Check sheet for the modelled part. Datum: model origin and axes. Units: mm. Round coordinates to 2 decimals unless told otherwise and drop trailing zeros. Order: outer loops, then holes, each group sorted by start corner. A loop starts at its lowest first (then second) coordinate and runs counter-clockwise, first axis right, second up.
```python
from build123d import *

# Parameters (mm, degrees)
SKETCH1_W                    = 220
SKETCH1_H                    = 560
BASE_FLANGE1_DEPTH           = 1.2
EDGE_FLANGE1_STRIP_W         = 8.2
EDGE_FLANGE1_STRIP_H         = 1.2
EDGE_FLANGE1_STRIP_CUT_DEPTH = 202.5
EDGE_FLANGE1_DEPTH           = 202.5
FILLET1_R                    = 1.5
SKETCH6_R                    = 2
CUT_EXTRUDE1_DEPTH           = 10
CUT_EXTRUDE2_DEPTH           = 10
LPATTERN1_COUNT              = 15
LPATTERN1_PITCH              = 7.2
FILLET2_R                    = 1.5


# Sheet-metal steps are written as plain solids
with BuildPart() as part:
    # Sketch1 → Base-Flange1 (new body)
    with BuildSketch(Plane(origin=(0, 0, 0), x_dir=(1, 0, 0), z_dir=(0, 1, 0))):
        with Locations((110, 280)):
            Rectangle(SKETCH1_W, SKETCH1_H)
    extrude(amount=BASE_FLANGE1_DEPTH)

    # Edge-Flange1 strip (across the edge) → Edge-Flange1 strip cut (cut)
    with BuildSketch(Plane(origin=(202.5, 0, 0), x_dir=(0, 0, -1), z_dir=(-1, 0, 0))):
        with Locations((-1.2, -0.6)):
            Rectangle(EDGE_FLANGE1_STRIP_W, EDGE_FLANGE1_STRIP_H)
    extrude(amount=EDGE_FLANGE1_STRIP_CUT_DEPTH, mode=Mode.SUBTRACT)

    # Edge-Flange1 section (across the edge) → Edge-Flange1 (add)
    with BuildSketch(Plane(origin=(202.5, 0, 0), x_dir=(0, 0, -1), z_dir=(-1, 0, 0))):
        with BuildLine():
            Line((0, 1.7), (0, 6.3))
            Line((0, 6.3), (1.2, 6.3))
            Line((1.2, 6.3), (1.2, 1.7))
            ThreePointArc((1.2, 1.7), (1.697918472, 0.497918472), (2.9, 0))
            Line((2.9, 0), (2.9, -1.2))
            ThreePointArc((2.9, -1.2), (0.849390335, -0.350609665), (0, 1.7))
        make_face()
    extrude(amount=EDGE_FLANGE1_DEPTH)

    # Fillet1
    fillet1_edges = [part.edges().sort_by_distance(p)[0] for p in [
        (202.5, -6.3, -0.6),
    ]]
    fillet(fillet1_edges, radius=FILLET1_R)

    # Sketch6 → Cut-Extrude1 (cut)
    with BuildSketch(Plane(origin=(0, 1.2, 0), x_dir=(1, 0, 0), z_dir=(0, 1, 0))):
        with Locations(Location((215.5, 531, 0), (0, 0, 270))):
            Circle(SKETCH6_R)
        with Locations(Location((215.5, 30, 0), (0, 0, 270))):
            Circle(SKETCH6_R)
        with Locations(Location((140, 555.5, 0), (0, 0, 270))):
            Circle(SKETCH6_R)
    extrude(amount=-CUT_EXTRUDE1_DEPTH, mode=Mode.SUBTRACT)

    # Sketch7 → Cut-Extrude2 (cut)
    with BuildSketch(Plane(origin=(0, 1.2, 0), x_dir=(1, 0, 0), z_dir=(0, 1, 0))):
        with BuildLine():
            Line((172.5, 477.1), (172.5, 512.9))
            ThreePointArc((172.5, 512.9), (174.6, 515), (176.7, 512.9))
            Line((176.7, 512.9), (176.7, 477.1))
            ThreePointArc((176.7, 477.1), (174.6, 475), (172.5, 477.1))
        make_face()
    cut_extrude2 = extrude(amount=-CUT_EXTRUDE2_DEPTH, mode=Mode.SUBTRACT)

    # LPattern1: Cut-Extrude2 ×15
    with Locations(*[(-i * LPATTERN1_PITCH, 0, 0) for i in range(1, LPATTERN1_COUNT)]):
        add(cut_extrude2, mode=Mode.SUBTRACT)

    # Fillet2
    fillet2_edges = [part.edges().sort_by_distance(p)[0] for p in [
        (220, 0.6, -560),
        (220, 0.6, 0),
    ]]
    fillet(fillet2_edges, radius=FILLET2_R)

    # Mirror1: part across plane


with BuildPart() as part_1:
    add(part.part)
    add(part.part.mirror(Plane(origin=(0, 1.2, 0), x_dir=(0, 0, 1), z_dir=(1, 0, 0))))


solid = part_1.part
```
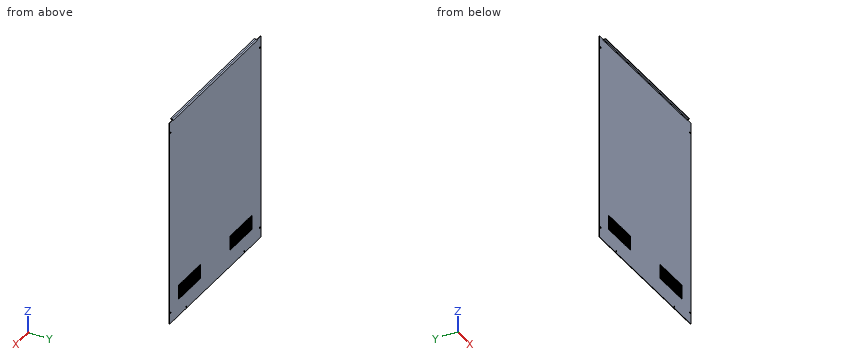
Item 1: Scan lines: line 1 along X through (y, z) = (0.45, -531); line 2 along Z through (x, y) = (-215.5, 0.4); line 3 along Z through (x, y) = (-140, 0.3). Record each from-to range of solid material in increasing order.
Answer:
line 1: x = -220 to -217.5, -213.5 to 213.5, 217.5 to 220
line 2: z = -560 to -533, -529 to -32, -28 to 0
line 3: z = -560 to -557.5, -553.5 to -514.47, -475.53 to -0.8
Item 2: Go/stop test with flat-tipped pins: P1, Ø1.4, axis at y = -3, z = -1, coming from the -X side; P2, Ø3, axis at x = -215.5, z = -531, coming from the -Y side; P3, Ø4, axis at x = -46.5, z = -117, coming from the -Y side. Record where each tip stops, or that it passes through.
Answer:
P1: stops at x = -202.5
P2: passes through
P3: stops at y = 0
Item 3: Sectioned sample at A-A (z = -378). Record the cut outline in (x, y), and give its area (3 significant figures).
Answer:
outline: (-220, 0) - (220, 0) - (220, 1.2) - (-220, 1.2) - close
area: 528 mm2
